Autodesk Inventor part; units mm, degrees
ref_plane "YZ Plane" through (0, 0, 0) normal (1, 0, 0) x (0, 1, 0)
ref_plane "XZ Plane" through (0, 0, 0) normal (0, 1, 0) x (-1, 0, 0)
ref_plane "XY Plane" through (0, 0, 0) normal (0, 0, 1) x (1, 0, 0)
sketch "Sketch1" plane through (0, 0, 0) normal (0, 0, 1) x (1, 0, 0)
  line L0 (-22.5, -22.5) -> (22.5, -22.5)
  line L1 (22.5, -22.5) -> (22.5, 22.5)
  line L2 (22.5, 22.5) -> (-22.5, 22.5)
  line L3 (-22.5, 22.5) -> (-22.5, -22.5)
  line L4 (-22.5, -22.5) -> (22.5, 22.5) construction
  line L5 (22.5, -22.5) -> (-22.5, 22.5) construction
  circle A0 centre (0, 0) radius 11
  line L6 (0, 0) -> (0, 17)
  line L7 (0, 0) -> (15.6, -9.0067)
  line L8 (0, 0) -> (-15.6, -9.0067)
  circle A1 centre (0, 17) radius 2.6
  circle A2 centre (15.6, -9.0067) radius 2.6
  circle A3 centre (-15.6, -9.0067) radius 2.6
  point P0 (22.5, -11.0947)
  point P1 (-22.5, -11.0947)
  dimension "d0" = 45
  dimension "d1" = 45
  dimension "d2" = 22
  dimension "d3" = 17
  dimension "d4" = 15.6
  dimension "d5" = 120
  dimension "d6" = 15.6
  dimension "d7" = 120
  dimension "d8" = 5.2
  dimension "d9" = 5.2
  dimension "d10" = 5.2
extrude "Extrusion2" add sketch "Sketch1" against normal blind 5
sketch "Sketch16" plane through (0, 0, 0) normal (0, 0, 1) x (1, 0, 0)
  line L0 (0, 0) -> (0, -32)
  line L1 (22.5, -22.5) -> (-22.5, -22.5)
  line L2 (-22.5, -22.5) -> (22.5, -22.5)
  line L3 (22.5, -22.5) -> (22.5, -32)
  line L4 (22.5, -32) -> (-22.5, -32)
  line L5 (-22.5, -32) -> (-22.5, -22.5)
  dimension "d37" = 32
extrude "Extrusion9" add sketch "Sketch16" along normal blind 12 and the other way blind 17
sketch "Sketch17" plane through (-22.5, -22.5, 0) normal (0, 1, 0) x (1, 0, 0)
  circle A0 centre (22.5, -6) radius 3.1
  circle A1 centre (22.5, -6) radius 5
  circle A2 centre (22.5, 11) radius 3.1
  circle A3 centre (22.5, 11) radius 5
  point P0 (22.5, 0)
  dimension "d42" = 6.2
  dimension "d43" = 10
  dimension "d44" = 6.2
  dimension "d45" = 10
extrude "Extrusion10" cut sketch "Sketch17" against normal through all contours A0 | A2
extrude "Extrusion11" cut sketch "Sketch17" against normal blind 5
equation "\"d1\" = d0"
equation "\"d4\" = d6"
equation "\"d7\" = d5"
equation "\"d9\" = d8"
equation "\"d10\" = d8"
properties part number "mount_v11"
Design review of the part built by this model. Coordinates are the model's own, in mm. A direction names the side the tool comes from. Round coordinates to 2 decimals unless told otherwise and drop trailing zeros. Order: outer loops, then holes, each group sorted by start corner. A loop starts at its lowest first (then second) coordinate and runs counter-clockwise, first axis right, second up. Notation, with made-up numbers: (73.5, 61.5) - (85.5, 61.5) arc R18 ccw to (85.5, 70.5) - close; hole circle Ø1 at (12.25, 23.5). An arc over 180 degrees is marked (long way). Return JSON: item names as keys, results as strings.
Q1. The part is to be moulded in two halves that separate along X. For faces 1 (the flat face through (5.3, -22.5, 5.9)), 2 (the cylindrical face through (-0.651, -24.965, -15.957)), 3 (the flat face through (-22.5, -15, -1)), say which applies: pulls with the +X half, pulls with the -X half, needs draft (parallel to the pull), parting line crosses it, or undercut.
Computed values:
{"face 1": "needs draft", "face 2": "undercut", "face 3": "pulls with the -X half"}
Q2. Consider section D-D on x = 15.6. Write out the cut boundary in (y, z).
Computed values:
{"outline": "(-32, -17) - (-22.5, -17) - (-22.5, -5) - (-11.61, -5) - (-11.61, 0) - (-22.5, 0) - (-22.5, 12) - (-32, 12) - close; (-6.41, -5) - (22.5, -5) - (22.5, 0) - (-6.41, 0) - close"}
Q3. Consider section C-C on z = 6. Write out the cut boundary in (x, y).
Computed values:
{"outline": "(-22.5, -32) - (-3.1, -32) - (-3.1, -27.5) - (-5, -27.5) - (-5, -22.5) - (-22.5, -22.5) - close; (3.1, -32) - (22.5, -32) - (22.5, -22.5) - (5, -22.5) - (5, -27.5) - (3.1, -27.5) - close"}
Q4. Wall thickness on L1, parallel to Y at x = 0, z = -4; L2, parallel to X at y = -26.25, z = 6; L3, parallel to X at y = 0, z = -1.55: over which ranges is each line inside the solid? List them lowest first. Write a range as [from, to].
Computed values:
{"L1": "y = [-32, -11], [11, 14.4], [19.6, 22.5]", "L2": "x = [-22.5, -5], [5, 22.5]", "L3": "x = [-22.5, -11], [11, 22.5]"}
Q5. Consider section A-A on y = 17. Write out the cut boundary in (x, z).
Computed values:
{"outline": "(-22.5, -5) - (-2.6, -5) - (-2.6, 0) - (-22.5, 0) - close; (2.6, -5) - (22.5, -5) - (22.5, 0) - (2.6, 0) - close"}
Q6. Machinability: for faces 4 (the flat face through (-5, 10, 0)), 5 (the flat face through (5.3, -22.5, -11.1)), 6 (the cylindrical face through (-4, -25, 9)), which of the approach directions +Z, -Z, +X, -X, +Y, -Y give a long, thin tool a straight path to every point of the face, cutting with its end or side? Answer none if there is none.
Computed values:
{"face 4": "+Z, +X, -X, +Y", "face 5": "-Z, +X, -X, +Y", "face 6": "+Y"}
Q7. For pin 1 Ø13.5 at (x, y) = (7.5, 2) entering from +Z; pin 2 Ø8 at (x, z) = (-2, -13.5) entering from +Y; pin 3 Ø1.5 at (x, y) = (-13.5, 17) entering from -Z, all flat-tipped, find the tip position at first contact; note any pin that passes through.
Computed values:
{"pin 1": "stops at z = 0", "pin 2": "stops at y = -22.5", "pin 3": "stops at z = -5"}
Q8. Consider section B-B on x = 0. Give the number of separate pieces and of enclosed holes in the cut face, plus the area to 3 significant figures.
Computed values:
{"separate pieces": "5", "enclosed holes": "0", "area": "209 mm2"}
